The model under review builds one solid part; all positions refer to its coordinate system, in mm. Face numbers are marked on the shaded views. A direction names the side the tool comes from. Coordinates: 2 decimals unless noted, no trailing zeros. Write each loop counter-clockwise with the first axis right and the second up, starting at its lowest first coordinate (ties: lowest second). Pieces come first, ordered by that corner, then holes. Notation, with made-up numbers: (55, -13) - (95, -13) arc R16 ccw to (95, -8) - close; hole circle Ø7 at (-34.75, 7). An arc over 180 degrees is marked (long way). Answer as CSV lines item,"result". Start each with the question number.
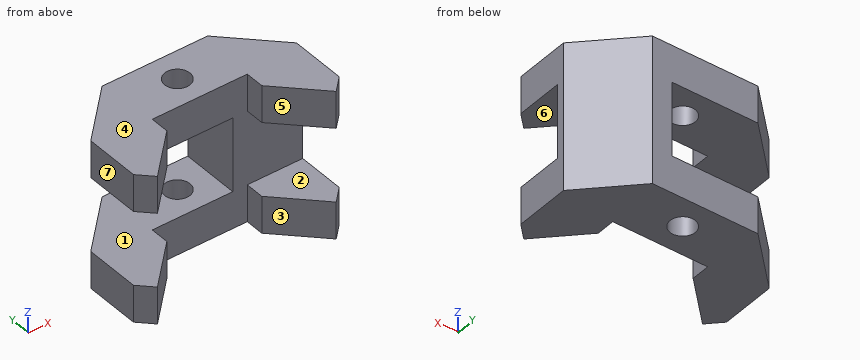
```python
from build123d import *

# Parameters (mm, degrees)
SKETCH_1_R          = 4.781543069
EXTRUDE_1_DEPTH     = 28
SKETCH_2_W          = 51.5
SKETCH_2_H          = 28
CUT_EXTRUDE_1_DEPTH = 45.997474683
SKETCH_3_W          = 28
SKETCH_3_H          = 23.235817225
CUT_EXTRUDE_2_DEPTH = 27.5


with BuildPart() as part:
    # 草图1 → 凸台-拉伸1 (new body, symmetric)
    with BuildSketch(Plane.XY):
        Polygon((0, 0), (-20, 0), (-39, -19), (-39, -39.882250994), (-33.884776311, -44.997474683), (-18, -29.112698372), (-18, -22), (18, -22), (18, -29.112698372), (33.884776311, -44.997474683), (39, -39.882250994), (39, -19), (20, 0), align=None)
        with Locations((0, -11)):
            Circle(SKETCH_1_R, mode=Mode.SUBTRACT)
    extrude(amount=EXTRUDE_1_DEPTH, both=True)

    # 草图2 → 切除-拉伸1 (cut, through all)
    with BuildSketch(Plane(origin=(0, 0, 0), x_dir=(1, 0, 0), z_dir=(0, 1, 0))):
        with Locations((-13.25, 0)):
            Rectangle(SKETCH_2_W, SKETCH_2_H)
    extrude(amount=-CUT_EXTRUDE_1_DEPTH, mode=Mode.SUBTRACT)

    # 草图3 → 切除-拉伸2 (cut, through all)
    with BuildSketch(Plane.ZY.offset(-12.5)):
        with Locations((0, -33.617908613)):
            Rectangle(SKETCH_3_W, SKETCH_3_H)
    extrude(amount=-CUT_EXTRUDE_2_DEPTH, mode=Mode.SUBTRACT)


solid = part.part
```
(1) Add section A-A on y = -11. Give the boundary of the cut face in (x, z).
(2) Add section C-C on z = 18.5. Give the boundary of the cut face in (x, y).
(3) For pin 1 (1 mm diameter, centred on y = -18, z = -15, fed in from +X); pin 2 (8 mm diameter, centred on x = -16.5, z = -6.5, fed in from +Y); pin 3 (1.5 mm diameter, centred on x = -13, z = -15, fed in from -Y); pin 4 (4 mm diameter, centred on y = -13.5, z = 3.5, fed in from -X), all flat-tipped, find the tip position at first contact; note any pin that passes through.
(4) Add section B-B on x = 0. Give the boundary of the cut face in (y, z).
(5) Add section D-D on z = 9.5. Give the boundary of the cut face in (x, y), then the cut area to 4 significant figures.
(6) The part is to be moulded in two halves that separate along X. For the marked faces 5, 6 and 7, say which applies: released by +X, released by -X, zero draft, split by the parting line, or undercut.
(7) Wall thickness on line 1 (Y direction, x = 0, z = -24); line 2 (Z direction, x = -11, y = -2); line 3 (X direction, y = -12.5, z = 22.5): over which ranges is each line inside the solid? List them lowest first.
(8) For the marked faces 1, 2, 3 and 4, list the 3-axis set-ups (+Z, -Z, +X, -X, +Y, -Y) from which the entire face can be reached by the end or side of a thin tool; tool diameter is ignored.
Reported:
1,outline,"(-31, -28) - (-4.78, -28) - (-4.78, -14) - (-31, -14) - close; (-31, 14) - (-4.78, 14) - (-4.78, 28) - (-31, 28) - close; (4.78, -28) - (31, -28) - (31, 28) - (4.78, 28) - (4.78, 14) - (12.5, 14) - (12.5, -14) - (4.78, -14) - close"
2,outline,"(-39, -39.88) - (-33.88, -45) - (-18, -29.11) - (-18, -22) - (18, -22) - (18, -29.11) - (33.88, -45) - (39, -39.88) - (39, -19) - (20, 0) - (-20, 0) - (-39, -19) - close; hole circle Ø9.56 at (0, -11)"
3,pin 1,"x = 38.5"
3,pin 2,"through"
3,pin 3,"y = -22"
3,pin 4,"x = 12.5"
4,outline,"(-22, -28) - (-15.78, -28) - (-15.78, -14) - (-22, -14) - close; (-22, 14) - (-15.78, 14) - (-15.78, 28) - (-22, 28) - close; (-6.22, -28) - (0, -28) - (0, -14) - (-6.22, -14) - close; (-6.22, 14) - (0, 14) - (0, 28) - (-6.22, 28) - close"
5,outline,"(12.5, -22) - (39, -22) - (39, -19) - (20, 0) - (12.5, 0) - close"
5,area,"402.5 mm²"
6,face 5,"undercut"
6,face 6,"zero draft"
6,face 7,"released by -X"
7,line 1,"-22 to -15.78, -6.22 to 0"
7,line 2,"-28 to -14, 14 to 28"
7,line 3,"-32.5 to -4.54, 4.54 to 32.5"
8,face 1,"-X, +Y, -Y"
8,face 2,"+X, -X, -Y"
8,face 3,"+Z, -Z, -Y"
8,face 4,"+Z, +X, -X, +Y, -Y"
